Read the model definition and answer for the solid it produces. Units are mm, in the model's axes. A direction names the side the tool comes from. Coordinates: 2 decimals unless noted, no trailing zeros. Loops run counter-clockwise (first coordinate to the right, second up) from the corner with the lowest first, then second, coordinate; pieces in that order, holes last.
Q1. Flat-ended cylindrical pins translate along their axes: P1, Ø3, axis at y = -0.5, z = 320, coming from the -X side; P2, Ø5.5, axis at y = 12, z = 290, coming from the +X side; P3, Ø1.8, axis at y = -18.5, z = 302, coming from the +X side. Find the tip coordinate at first contact, or state that the pin passes through.
Q2. Section D-D (y = -9) is taken. Give the vertices of the cut face in (x, z).
Q3. Section C-C (z = 312) is taken. Give the vertices of the cut face in (x, y), then the cut area to 3 significant figures.
Q4. Straight lines are drawn through the part: line 1 (Y direction, x = 195.15, z = 312); line 2 (Z direction, x = 195.2, y = -12); line 3 (Z direction, x = 219.5, y = 13). For each, find the intervals that lie inside material, in ascending order.
Q5. Section A-A (x = 212.5) is taken. Give the vertices of the cut face in (y, z), then the cut area to 3 significant figures.
Q6. The mould has two halves that part along X. Classify faces 5 (the face through (213.25, 0, 283)), 6 (the face through (221, 0, 321)), 7 (the face through (202, 19.5, 302)): pulls with the +X half, pulls with the -X half, needs draft (parallel to the pull), parting line crosses it, or undercut.
Q7. Which of the six approach directions +Z, -Z, +X, -X, +Y, -Y give full straight-line access (tool end or side, diameter ignored) to faces 1 (the face through (212, 0, 320.7)), 2 (the face through (198, 5, 322.3)), 3 (the face through (217, 0, 318.3)), 4 (the face through (203, 17.2, 301))?
Q8. Section B-B (y = -4) is taken. Give the vertices of the cut face in (x, z).
from build123d import *

# Parameters (mm, degrees)
SKETCH1_W           = 42.6
SKETCH1_H           = 39
BOSS_EXTRUDE1_DEPTH = 2.7
SKETCH2_W           = 42.6
SKETCH2_H           = 2.3
BOSS_EXTRUDE2_DEPTH = 12.7
SKETCH3_W           = 4
SKETCH3_H           = 39
BOSS_EXTRUDE3_DEPTH = 18.4
SKETCH4_R           = 1.7
SKETCH4_W           = 33.2
SKETCH4_H           = 13
CUT_EXTRUDE1_DEPTH  = 2.7
SKETCH5_W           = 4.7
SKETCH5_H           = 6
CUT_EXTRUDE2_DEPTH  = 2.4
SKETCH6_W           = 2.5
SKETCH6_H           = 2.4
CUT_EXTRUDE3_DEPTH  = 30
SKETCH7_W           = 5.9
SKETCH7_H           = 39
SKETCH7_W_2         = 4
BOSS_EXTRUDE4_DEPTH = 6
BOSS_EXTRUDE5_DEPTH = 1.9
CUT_EXTRUDE4_DEPTH  = 326.914559356


with BuildPart() as part:
    # Sketch1 → Boss-Extrude1 (new body)
    with BuildSketch(Plane(origin=(193.9, 0, 0), x_dir=(0, 0, -1), z_dir=(1, 0, 0))):
        with Locations((-301, 0)):
            Rectangle(SKETCH1_W, SKETCH1_H)
    extrude(amount=BOSS_EXTRUDE1_DEPTH)

    # Sketch2 → Boss-Extrude2 (add)
    with BuildSketch(Plane(origin=(196.6, 0, 0), x_dir=(0, 0, -1), z_dir=(1, 0, 0))):
        with Locations((-301, 18.35)):
            Rectangle(SKETCH2_W, SKETCH2_H)
        with Locations((-301, -18.35)):
            Rectangle(SKETCH2_W, SKETCH2_H)
    extrude(amount=BOSS_EXTRUDE2_DEPTH)

    # Sketch3 → Boss-Extrude3 (add)
    with BuildSketch(Plane(origin=(196.6, 0, 0), x_dir=(0, 0, -1), z_dir=(1, 0, 0))):
        with Locations((-320.3, 0)):
            Rectangle(SKETCH3_W, SKETCH3_H)
        with Locations((-281.7, 0)):
            Rectangle(SKETCH3_W, SKETCH3_H)
    extrude(amount=BOSS_EXTRUDE3_DEPTH)

    # Sketch4 → Cut-Extrude1 (cut)
    with BuildSketch(Plane(origin=(193.9, 0, 0), x_dir=(0, 0, -1), z_dir=(1, 0, 0))):
        with Locations(Location((-290, 12, 0), (0, 0, 180))):
            Circle(SKETCH4_R)
        with Locations(Location((-290, -12, 0), (0, 0, 180))):
            Circle(SKETCH4_R)
        with Locations(Location((-312, 12, 0), (0, 0, 180))):
            Circle(SKETCH4_R)
        with Locations(Location((-312, -12, 0), (0, 0, 180))):
            Circle(SKETCH4_R)
        with Locations((-306.4, 0)):
            Rectangle(SKETCH4_W, SKETCH4_H)
    extrude(amount=CUT_EXTRUDE1_DEPTH, mode=Mode.SUBTRACT)

    # Sketch5 → Cut-Extrude2 (cut)
    with BuildSketch(Plane(origin=(196.6, 0, 0), x_dir=(0, 0, -1), z_dir=(1, 0, 0))):
        with Locations((-320.65, 0)):
            Rectangle(SKETCH5_W, SKETCH5_H)
    extrude(amount=CUT_EXTRUDE2_DEPTH, mode=Mode.SUBTRACT)

    # Sketch6 → Cut-Extrude3 (cut, symmetric)
    with BuildSketch(Plane(origin=(0, 0, 0), x_dir=(1, 0, 0), z_dir=(0, 1, 0))):
        with Locations((212, -319.5)):
            Rectangle(SKETCH6_W, SKETCH6_H)
        with Locations((212, -282.5)):
            Rectangle(SKETCH6_W, SKETCH6_H)
    extrude(amount=CUT_EXTRUDE3_DEPTH, both=True, mode=Mode.SUBTRACT)

    # Sketch7 → Boss-Extrude4 (add)
    with BuildSketch(Plane(origin=(215, 0, 0), x_dir=(0, 0, -1), z_dir=(1, 0, 0))):
        with Locations((-321.25, 0)):
            Rectangle(SKETCH7_W, SKETCH7_H)
        with Locations((-281.7, 0)):
            Rectangle(SKETCH7_W_2, SKETCH7_H)
    extrude(amount=BOSS_EXTRUDE4_DEPTH)

    # Sketch8 → Boss-Extrude5 (add)
    with BuildSketch(Plane.XY.offset(322.3)):
        Polygon((193.9, -19.5), (215, -19.5), (215, 19.5), (193.9, 19.5), (193.9, 6.5), (199, 6.5), (199, -6.5), (193.9, -6.5), align=None)
    extrude(amount=BOSS_EXTRUDE5_DEPTH)

    # Sketch9 → Cut-Extrude4 (cut, through all)
    with BuildSketch(Plane(origin=(193.9, 0, 0), x_dir=(0, 0, -1), z_dir=(1, 0, 0))):
        with BuildLine():
            Line((-324.2, 13.5), (-325.5, 13.5))
            Line((-325.5, 13.5), (-325.5, 20.5))
            Line((-325.5, 20.5), (-318.2, 20.5))
            Line((-318.2, 20.5), (-318.2, 19.5))
            ThreePointArc((-318.2, 19.5), (-322.442640687, 17.742640687), (-324.2, 13.5))
        make_face()
        with BuildLine():
            Line((-324.2, -13.5), (-325.5, -13.5))
            Line((-325.5, -13.5), (-325.5, -20.5))
            Line((-325.5, -20.5), (-318.2, -20.5))
            Line((-318.2, -20.5), (-318.2, -19.5))
            ThreePointArc((-318.2, -19.5), (-322.442640687, -17.742640687), (-324.2, -13.5))
        make_face()
        with BuildLine():
            Line((-279.7, 13.5), (-278.4, 13.5))
            Line((-278.4, 13.5), (-278.4, 20.5))
            Line((-278.4, 20.5), (-285.7, 20.5))
            Line((-285.7, 20.5), (-285.7, 19.5))
            ThreePointArc((-285.7, 19.5), (-281.457359313, 17.742640687), (-279.7, 13.5))
        make_face()
        with BuildLine():
            Line((-279.7, -13.5), (-278.4, -13.5))
            Line((-278.4, -13.5), (-278.4, -20.5))
            Line((-278.4, -20.5), (-285.7, -20.5))
            Line((-285.7, -20.5), (-285.7, -19.5))
            ThreePointArc((-285.7, -19.5), (-281.457359313, -17.742640687), (-279.7, -13.5))
        make_face()
    extrude(amount=CUT_EXTRUDE4_DEPTH, mode=Mode.SUBTRACT)


solid = part.part
Numbers:
1. P1: stops at x = 199
1. P2: stops at x = 196.6
1. P3: stops at x = 209.3
2. outline: (193.9, 279.7) - (221, 279.7) - (221, 283.7) - (213.25, 283.7) - (213.25, 281.3) - (210.75, 281.3) - (210.75, 283.7) - (196.6, 283.7) - (196.6, 318.3) - (210.75, 318.3) - (210.75, 320.7) - (213.25, 320.7) - (213.25, 318.3) - (221, 318.3) - (221, 324.2) - (193.9, 324.2) - close
3. outline: (193.9, -19.5) - (209.3, -19.5) - (209.3, -17.2) - (196.6, -17.2) - (196.6, -13.7) - (193.9, -13.7) - close; (193.9, -10.3) - (196.6, -10.3) - (196.6, -6.5) - (193.9, -6.5) - close; (193.9, 6.5) - (196.6, 6.5) - (196.6, 10.3) - (193.9, 10.3) - close; (193.9, 13.7) - (196.6, 13.7) - (196.6, 17.2) - (209.3, 17.2) - (209.3, 19.5) - (193.9, 19.5) - close
3. area: 110 mm2
4. line 1: y = -19.5 to -13.7, -10.3 to -6.5, 6.5 to 10.3, 13.7 to 19.5
4. line 2: z = 279.7 to 288.3, 291.7 to 310.3, 313.7 to 324.2
4. line 3: z = 279.7 to 283.7, 318.3 to 324.2
5. outline: (-18.95, 320.7) - (18.95, 320.7) arc R6 ccw to (13.5, 324.2) - (-13.5, 324.2) arc R6 ccw to start; (-17.58, 281.3) arc R6 ccw to (-13.5, 279.7) - (13.5, 279.7) arc R6 ccw to (17.58, 281.3) - close
5. area: 174 mm2
6. face 5: undercut
6. face 6: pulls with the +X half
6. face 7: needs draft
7. face 1: +Y, -Y
7. face 2: +Z, -X
7. face 3: +X, +Y, -Y
7. face 4: +X
8. outline: (193.9, 279.7) - (221, 279.7) - (221, 283.7) - (213.25, 283.7) - (213.25, 281.3) - (210.75, 281.3) - (210.75, 283.7) - (196.6, 283.7) - (196.6, 289.8) - (193.9, 289.8) - close; (196.6, 318.3) - (210.75, 318.3) - (210.75, 320.7) - (213.25, 320.7) - (213.25, 318.3) - (221, 318.3) - (221, 324.2) - (199, 324.2) - (199, 322.3) - (196.6, 322.3) - close
